```python
from build123d import *

# Parameters (mm, degrees)
SKETCH1_R           = 9.906
SKETCH1_R_2         = 14.2875
SKETCH1_R_3         = 2.667
BOSS_EXTRUDE1_DEPTH = 6.35


with BuildPart() as part:
    # Sketch1 → Boss-Extrude1 (new body)
    with BuildSketch(Plane.XY):
        Polygon((12.15597468, 91.000063132), (122.95536215, 62.928979497), (132.147395909, 47.498927153), (123.172465774, 12.073976179), (107.832275805, -3.691447117), (13.850085892, 20.118990589), (0.062035253, 43.264069106), align=None)
        with Locations((19.05, 54.027523873)):
            Circle(SKETCH1_R, mode=Mode.SUBTRACT)
        with Locations((106.981625, 31.75)):
            Circle(SKETCH1_R_2, mode=Mode.SUBTRACT)
        with Locations((106.981625, 57.15)):
            Circle(SKETCH1_R_3, mode=Mode.SUBTRACT)
        with Locations((106.981625, 6.35)):
            Circle(SKETCH1_R_3, mode=Mode.SUBTRACT)
        with Locations((19.05, 79.427523873)):
            Circle(SKETCH1_R_3, mode=Mode.SUBTRACT)
        with Locations((19.05, 28.627523873)):
            Circle(SKETCH1_R_3, mode=Mode.SUBTRACT)
    extrude(amount=BOSS_EXTRUDE1_DEPTH)


solid = part.part
```
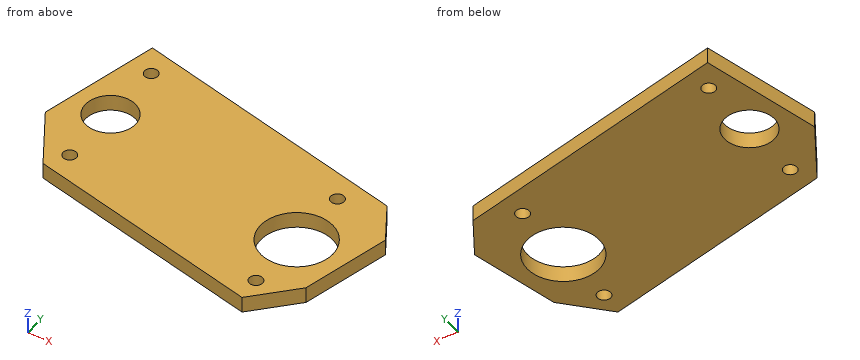
Input: part model. Units: mm. Frame: model coordinates. Round coordinates to 2 decimals unless told otherwise and drop trailing zeros. Loops run counter-clockwise (first coordinate to the right, second up) from the corner with the lowest first, then second, coordinate; pieces in that order, holes last. Notation, with made-up numbers: (3, 25) -> (62, 25) arc R21 cw to (62, 36) -> close; hole circle Ø5 at (-12, 56). An arc over 180 degrees is marked (long way). One line per item, written item: value.
(1) Section A-A (x = 106.5). Return the cut outline in (y, z), plus the area to 3 significant figures.
Geometry check:
outline: (-3.35, 0) -> (3.73, 0) -> (3.73, 6.35) -> (-3.35, 6.35) -> close; (8.97, 0) -> (17.47, 0) -> (17.47, 6.35) -> (8.97, 6.35) -> close; (46.03, 0) -> (54.53, 0) -> (54.53, 6.35) -> (46.03, 6.35) -> close; (59.77, 0) -> (67.1, 0) -> (67.1, 6.35) -> (59.77, 6.35) -> close
area: 199 mm2
(2) Section C-C (y = 39). Return the cut outline in (x, z).
Geometry check:
outline: (2.6, 0) -> (94.67, 0) -> (94.67, 6.35) -> (2.6, 6.35) -> close; (119.29, 0) -> (129.99, 0) -> (129.99, 6.35) -> (119.29, 6.35) -> close
(3) Material intervals for line 1 (X direction, y = 59.5, z = 1.75); line 2 (Y direction, x = 105, z = 1); line 3 (Y direction, x = 108.5, z = 2.75), sorted ascending. Write a range as [from, to].
Geometry check:
line 1: [4.18, 10.79], [27.31, 105.72], [108.24, 125]
line 2: [-2.97, 4.57], [8.13, 17.6], [45.9, 55.37], [58.93, 67.48]
line 3: [-3.01, 4.16], [8.54, 17.54], [45.96, 54.96], [59.34, 66.59]
(4) Section B-B (y = 57.15). Return the cut outline in (x, z).
Geometry check:
outline: (3.58, 0) -> (9.65, 0) -> (9.65, 6.35) -> (3.58, 6.35) -> close; (28.45, 0) -> (104.31, 0) -> (104.31, 6.35) -> (28.45, 6.35) -> close; (109.65, 0) -> (126.4, 0) -> (126.4, 6.35) -> (109.65, 6.35) -> close
(5) Pin query (flat end, axial travel): pin 1 (3 mm diameter, centred on x = 106.98, y = 57.15, fed in from -Z); pin 2 (1 mm diameter, centred on x = 46, z = 1.5, fed in from -Y). Return the tip coordinate at first contact, or that it passes through.
Geometry check:
pin 1: through
pin 2: y = 11.85
(6) Section D-D (z = 1.25). Give the number of separate pieces and of enclosed holes in the cut face, plus the area to 3 significant figures.
Geometry check:
separate pieces: 1
enclosed holes: 6
area: 7,270 mm2
